Here's how the part is built. I have some questions about the finished solid (model axes, mm). Give positions to 0.01 mm unless a question says otherwise; leave off trailing zeros. Order: outer loops, then holes, each group sorted by start corner. A loop starts at its lowest first (then second) coordinate and runs counter-clockwise, first axis right, second up.
Autodesk Inventor part; units mm, degrees
ref_plane "YZ Plane" through (0, 0, 0) normal (1, 0, 0) x (0, 1, 0)
ref_plane "XZ Plane" through (0, 0, 0) normal (0, 1, 0) x (-1, 0, 0)
ref_plane "XY Plane" through (0, 0, 0) normal (0, 0, 1) x (1, 0, 0)
sketch "Sketch1" plane through (0, 0, 0) normal (0, 0, 1) x (1, 0, 0)
  line L0 (300, 0) -> (300, -90)
  line L1 (300, -90) -> (0, -90)
  line L2 (67.6148, -18.1173) -> (23.6156, -182.3247)
  line L3 (23.6156, -182.3247) -> (-43.9992, -164.2074)
  line L4 (-43.9992, -164.2074) -> (0, 0)
  line L5 (0, 0) -> (67.6148, -18.1173)
  line L6 (0, 0) -> (300, 0)
  line L7 (0, -90) -> (0, 0)
  dimension "d0" = 300
  dimension "d1" = 90
  dimension "d2" = 70
  dimension "d3" = 170
  dimension "d5" = 105
  dimension "d6" = 0
  dimension "d7" = 0
  dimension "d8" = 0
  dimension "d9" = 300
extrude "Extrusion1" add sketch "Sketch1" along normal blind 10
sketch "Sketch2" plane through (0, 0, 10) normal (0, 0, 1) x (1, 0, 0)
  line L0 (300, -90) -> (300, 0)
  line L1 (300, -20) -> (300, -60)
  line L2 (23.6156, -182.3247) -> (48.3539, -90)
  line L3 (48.3539, -90) -> (300, -60)
  line L4 (300, -20) -> (250, -20)
  line L5 (250, -20) -> (118.443, 27.8828)
  line L6 (48.3539, -90) -> (300, -90)
  line L7 (48.3539, -90) -> (300, -90)
  line L8 (300, -90) -> (300, -60)
  line L9 (300, 0) -> (0, 0)
  line L10 (195.0505, 0) -> (300, 0)
  line L11 (300, 0) -> (300, -20)
  dimension "d12" = 40
  dimension "d13" = 20
  dimension "d14" = 50
  dimension "d15" = 140
  dimension "d16" = 160
extrude "Extrusion2" cut sketch "Sketch2" against normal blind 10
properties part number "Pivot Link"
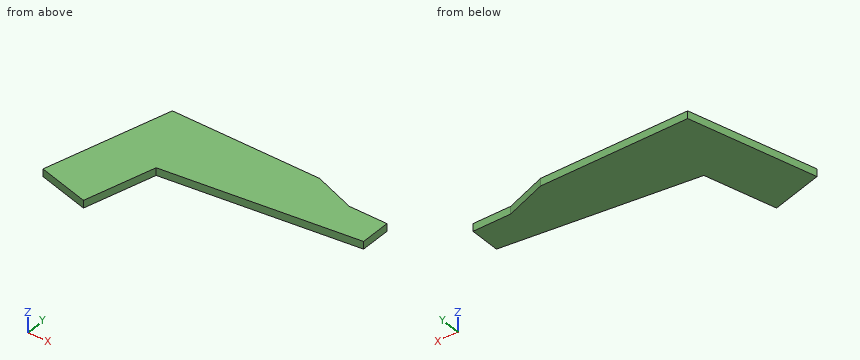
Q1. I need wall thicknesses on L1, parallel to Y at x = 86, z = 6.75; L2, parallel to X at y = -38, z = 3; L3, parallel to Y at x = 134, z = 8.25. Which ranges of each line are inside material? Lowest first, please.
Filled sheet:
L1: y = -85.51 to 0
L2: x = -10.18 to 300
L3: y = -79.79 to 0
Q2. If we section it at B-B on x = 124: List the corners of the cut face in (y, z) for me.
Filled sheet:
outline: (-80.98, 0) - (0, 0) - (0, 10) - (-80.98, 10) - close
Q3. If we section it at C-C on y = -115: List the corners of the cut face in (x, z) for me.
Filled sheet:
outline: (-30.81, 0) - (41.66, 0) - (41.66, 10) - (-30.81, 10) - close
Q4. If we section it at A-A on z = 5.5: List the corners of the cut face in (x, y) for me.
Filled sheet:
outline: (-44, -164.21) - (23.62, -182.32) - (48.35, -90) - (300, -60) - (300, -20) - (250, -20) - (195.05, 0) - (0, 0) - close
Q5. I'm going to push flat-ended pins straight in: P1, Ø5, axis at y = -163.5, z = 8, coming from the +X side; P2, Ø3, axis at x = 265, z = 4.5, coming from the +Y side; P3, Ø1.5, axis at y = -156.5, z = 6.5, coming from the +X side. Where does each tip first touch, or does it pass through?
Filled sheet:
P1: stops at x = 29.33
P2: stops at y = -20
P3: stops at x = 30.74
